Read the model definition and answer for the solid it produces. Units are mm, in the model's axes. A direction names the side the tool comes from. Give positions to 0.01 mm unless a question says otherwise; leave off trailing zeros. Loops run counter-clockwise (first coordinate to the right, second up) from the corner with the lowest first, then second, coordinate; pieces in that order, holes last. Notation, with made-up numbers: (-14.75, 36.25) - (29.25, 36.25) arc R29 cw to (29.25, 69.25) - close; hole circle Ø2 at (-2, -19.5). An arc over 180 degrees is marked (long way). Write item = value, one per line.
```python
from build123d import *

# Parameters (mm, degrees)
SKETCH2_W                = 90
SKETCH2_H                = 120
BOSS_EXTRUDE1_DEPTH      = 31.5
SKETCH4_W                = 87
SKETCH4_H                = 117
CUT_EXTRUDE1_DEPTH       = 30
FILLET4_R                = 4
SKETCH18_W               = 57
SKETCH18_H               = 53.6
KHAY_PIN_DEPTH           = 12.5
SKETCH21_W               = 53
SKETCH21_H               = 49.6
BOSS_EXTRUDE11_DEPTH     = 15
SKETCH22_W               = 53
SKETCH22_H               = 49.6
CUT_EXTRUDE4_DEPTH       = 13.5
SKETCH30_W               = 7
SKETCH30_H               = 14
CUT_EXTRUDE8_DEPTH       = 5
SKETCH34_R               = 4.242640687
BOSS_EXTRUDE12_DEPTH     = 7
SKETCH37_W               = 7.9
SKETCH37_H               = 15.9
CUT_EXTRUDE10_DEPTH      = 5
MIRROR2_COPY_1_SKETCH_R  = 4.242640687
MIRROR2_COPY_1_DEPTH     = 7
SKETCH38_R               = 10
CUT_EXTRUDE11_DEPTH      = 10
SKETCH40_W               = 6
SKETCH40_H               = 49.6
BOSS_EXTRUDE13_DEPTH     = 5.8
SKETCH48_W               = 71
SKETCH48_H               = 6
BOSS_EXTRUDE14_DEPTH     = 5.8
SKETCH50_W               = 2.3
SKETCH50_H               = 1.8
CUT_EXTRUDE14_DEPTH      = 49.6
SKETCH52_R               = 1.4
CUT_EXTRUDE15_DEPTH      = 10
MIRROR10_COPY_1_SKETCH_R = 1.4
MIRROR10_COPY_1_DEPTH    = 10
BOSS_EXTRUDE16_DEPTH     = 10


with BuildPart() as part:
    # Sketch2 → Boss-Extrude1 (new body)
    with BuildSketch(Plane.XY):
        Rectangle(SKETCH2_W, SKETCH2_H)
    extrude(amount=BOSS_EXTRUDE1_DEPTH)

    # Sketch4 → Cut-Extrude1 (cut)
    with BuildSketch(Plane.XY.offset(31.5)):
        Rectangle(SKETCH4_W, SKETCH4_H)
    extrude(amount=-CUT_EXTRUDE1_DEPTH, mode=Mode.SUBTRACT)

    # Fillet4
    fillet4_edges = [part.edges().sort_by_distance(p)[0] for p in [
        (45, -60, 15.75),
        (-45, -60, 15.75),
        (-45, 60, 15.75),
        (45, 60, 15.75),
    ]]
    fillet(fillet4_edges, radius=FILLET4_R)

    # Sketch18 → khay_pin (add)
    with BuildSketch(Plane.XY.offset(1.5)):
        with Locations((0, -21.775547075)):
            Rectangle(SKETCH18_W, SKETCH18_H)
    extrude(amount=KHAY_PIN_DEPTH)

    # Sketch21 → Boss-Extrude11 (add)
    with BuildSketch(Plane.XY.offset(14)):
        with Locations((0, -21.775547075)):
            Rectangle(SKETCH21_W, SKETCH21_H)
    extrude(amount=-BOSS_EXTRUDE11_DEPTH)

    # Sketch22 → Cut-Extrude4 (cut)
    with BuildSketch(Plane(origin=(0, 0, -1), x_dir=(-1, 0, 0), z_dir=(0, 0, -1))):
        with Locations((0, -21.775547075)):
            Rectangle(SKETCH22_W, SKETCH22_H)
    extrude(amount=-CUT_EXTRUDE4_DEPTH, mode=Mode.SUBTRACT)

    # Sketch30 → Cut-Extrude8 (cut)
    with BuildSketch(Plane.ZY.offset(-26.5)):
        with Locations((9, -8.975547075)):
            Rectangle(SKETCH30_W, SKETCH30_H)
    extrude(amount=-CUT_EXTRUDE8_DEPTH, mode=Mode.SUBTRACT)

    # Sketch34 → Boss-Extrude12 (add)
    with BuildSketch(Plane.XY.offset(31.5)):
        with Locations((-40.5, 55.5)):
            Circle(SKETCH34_R)
    boss_extrude12 = extrude(amount=-BOSS_EXTRUDE12_DEPTH)

    # Sketch37 → Cut-Extrude10 (cut)
    with BuildSketch(Plane(origin=(45, 0, 0), x_dir=(0, 0, -1), z_dir=(1, 0, 0))):
        with Locations((-18.5, 28)):
            Rectangle(SKETCH37_W, SKETCH37_H)
    extrude(amount=-CUT_EXTRUDE10_DEPTH, mode=Mode.SUBTRACT)

    # Mirror1: Boss-Extrude12 across plane
    add(boss_extrude12.mirror(Plane(origin=(0, 0, 0), x_dir=(0, 0, 1), z_dir=(1, 0, 0))))

    # Mirror2: Boss-Extrude12 across plane
    add(boss_extrude12.mirror(Plane.ZX))

    # Mirror2 copy 1 sketch → Mirror2 copy 1 (add)
    with BuildSketch(Plane(origin=(0, 0, 31.5), x_dir=(-1, 0, 0), z_dir=(0, 0, 1))):
        with Locations((-40.5, 55.5)):
            Circle(MIRROR2_COPY_1_SKETCH_R)
    extrude(amount=-MIRROR2_COPY_1_DEPTH)

    # Sketch38 → Cut-Extrude11 (cut)
    with BuildSketch(Plane.XY.offset(14)):
        with Locations((0, -21.775547075)):
            Circle(SKETCH38_R)
    extrude(amount=-CUT_EXTRUDE11_DEPTH, mode=Mode.SUBTRACT)

    # Sketch40 → Boss-Extrude13 (add)
    with BuildSketch(Plane(origin=(0, 0, 0), x_dir=(-1, 0, 0), z_dir=(0, 0, -1))):
        with Locations((-32.5, -21.775547075)):
            Rectangle(SKETCH40_W, SKETCH40_H)
    boss_extrude13 = extrude(amount=BOSS_EXTRUDE13_DEPTH)

    # Mirror3: Boss-Extrude13 across plane
    add(boss_extrude13.mirror(Plane(origin=(0, 0, 0), x_dir=(0, 0, 1), z_dir=(1, 0, 0))))

    # Sketch48 → Boss-Extrude14 (add)
    with BuildSketch(Plane(origin=(0, 0, 0), x_dir=(-1, 0, 0), z_dir=(0, 0, -1))):
        with Locations((0, -49.575547075)):
            Rectangle(SKETCH48_W, SKETCH48_H)
    extrude(amount=BOSS_EXTRUDE14_DEPTH)

    # Sketch50 → Cut-Extrude14 (cut)
    with BuildSketch(Plane(origin=(0, 3.024452925, 0), x_dir=(1, 0, 0), z_dir=(0, 1, 0))):
        with Locations((30.65, 2.9)):
            Rectangle(SKETCH50_W, SKETCH50_H)
    cut_extrude14 = extrude(amount=-CUT_EXTRUDE14_DEPTH, mode=Mode.SUBTRACT)

    # Mirror7: Cut-Extrude14 across plane
    add(cut_extrude14.mirror(Plane(origin=(0, 0, 0), x_dir=(0, 0, 1), z_dir=(1, 0, 0))), mode=Mode.SUBTRACT)

    # Sketch52 → Cut-Extrude15 (cut)
    with BuildSketch(Plane.XY.offset(31.5)):
        with Locations((-39.939339828, 54.939339828)):
            Circle(SKETCH52_R)
    cut_extrude15 = extrude(amount=-CUT_EXTRUDE15_DEPTH, mode=Mode.SUBTRACT)

    # Mirror9: Cut-Extrude15 across plane
    add(cut_extrude15.mirror(Plane(origin=(0, 0, 0), x_dir=(0, 0, 1), z_dir=(1, 0, 0))), mode=Mode.SUBTRACT)

    # Mirror10: Cut-Extrude15 across plane
    add(cut_extrude15.mirror(Plane.ZX), mode=Mode.SUBTRACT)

    # Mirror10 copy 1 sketch → Mirror10 copy 1 (cut)
    with BuildSketch(Plane(origin=(0, 0, 31.5), x_dir=(-1, 0, 0), z_dir=(0, 0, 1))):
        with Locations((-39.939339828, 54.939339828)):
            Circle(MIRROR10_COPY_1_SKETCH_R)
    extrude(amount=-MIRROR10_COPY_1_DEPTH, mode=Mode.SUBTRACT)

    # Sketch51 → Boss-Extrude16 (add)
    with BuildSketch(Plane.XY.offset(1.5)):
        Polygon((43.5, -52.5), (37.5, -58.5), (43.5, -58.5), align=None)
    boss_extrude16 = extrude(amount=BOSS_EXTRUDE16_DEPTH)

    # Mirror11: Boss-Extrude16 across plane
    add(boss_extrude16.mirror(Plane(origin=(0, 0, 0), x_dir=(0, 0, 1), z_dir=(1, 0, 0))))


solid = part.part
```
1) A cutting plane is placed at C-C on x = 14. Determine the outline of the cut face in (y, z), then the cut area to 3 significant figures.
Output:
outline = (-60, 0) - (-52.58, 0) - (-52.58, -5.8) - (-46.58, -5.8) - (-46.58, 12.5) - (3.02, 12.5) - (3.02, 0) - (60, 0) - (60, 31.5) - (58.5, 31.5) - (58.5, 1.5) - (5.02, 1.5) - (5.02, 14) - (-48.58, 14) - (-48.58, 1.5) - (-58.5, 1.5) - (-58.5, 31.5) - (-60, 31.5) - close
area = 355 mm²
2) A cutting plane is placed at A-A on x = 0. Determine the outline of the cut face in (y, z).
Output:
outline = (-60, 0) - (-52.58, 0) - (-52.58, -5.8) - (-46.58, -5.8) - (-46.58, 12.5) - (-31.78, 12.5) - (-31.78, 14) - (-48.58, 14) - (-48.58, 1.5) - (-58.5, 1.5) - (-58.5, 31.5) - (-60, 31.5) - close; (-11.78, 12.5) - (3.02, 12.5) - (3.02, 0) - (60, 0) - (60, 31.5) - (58.5, 31.5) - (58.5, 1.5) - (5.02, 1.5) - (5.02, 14) - (-11.78, 14) - close
3) Each of these flat-tipped pins is pushed along its axis until it touches: P1, Ø3.5, axis at x = 41.5, y = -56, coming from the -Z side; P2, Ø0.6, axis at y = -28, z = -1, coming from the -X side; P3, Ø3, axis at x = -34, z = -2.5, coming from the +Y side. Where does it stop, or does it pass through?
Output:
P1 = 0
P2 = -35.5
P3 = 3.02
4) A tool of negligible diameter and unlimited length cuts with its end or side. For faces 5 (the face through (-42, 55, 24.5)), 6 (the face through (-26.5, -22, 6)), 7 (the face through (39.19, 56.12, 28.05)), 8 (the face through (35.5, -25, -3)), from which of +Z, -Z, +X, -X, +Y, -Y can it reach the whole face along a straight path? Write none if from no direction.
Output:
face_5 = none
face_6 = -Z
face_7 = +Z
face_8 = -Z, +X, +Y, -Y
5) A cutting plane is placed at B-B on y = 33.5. Determine the outline of the cut face in (x, z).
Output:
outline = (-45, 0) - (45, 0) - (45, 14.55) - (43.5, 14.55) - (43.5, 1.5) - (-43.5, 1.5) - (-43.5, 31.5) - (-45, 31.5) - close; (43.5, 22.45) - (45, 22.45) - (45, 31.5) - (43.5, 31.5) - close
6) Find the intervals of material crossed by probe 1 along X at (y, z) = (-41.5, 9.5); probe 2 along Y at (x, z) = (-20, 6.5); probe 3 along X at (y, z) = (-29.5, -3.5), in increasing order.
Output:
probe_1 = -45 to -43.5, -28.5 to -26.5, 26.5 to 28.5, 43.5 to 45
probe_2 = -60 to -58.5, -48.58 to -46.58, 3.02 to 5.02, 58.5 to 60
probe_3 = -35.5 to -31.8, 31.8 to 35.5
7) The mould has two halves that part along Y. Classify faces 1 (the face through (-1, -60, 16)), 2 (the face through (1, -33, 12.5)), 3 (the face through (-1, 14, 0)), 4 (the face through (-43.5, -1, 17)): pulls with the +Y half, pulls with the -Y half, needs draft (parallel to the pull), parting line crosses it, or undercut.
Output:
face_1 = pulls with the -Y half
face_2 = undercut
face_3 = needs draft
face_4 = undercut
